CAD build for the part. Positions are in the model's coordinates, mm. A direction names the side the tool comes from. Round coordinates to 2 decimals unless told otherwise and drop trailing zeros. Write each loop counter-clockwise with the first axis right and the second up, starting at its lowest first coordinate (ties: lowest second). Pieces come first, ordered by that corner, then holes. Notation, with made-up numbers: (-30.75, 16) - (24.25, 16) arc R27 cw to (24.25, 38) - close; hole circle Ø6 at (87.25, -2.5). An arc over 180 degrees is marked (long way). Put each result on its own line as item: value. Start each with the question number.
Item 1: Drill centre lines: line 1 (X direction, y = 6.25, z = 34); line 2 (X direction, y = 14.3, z = 250); line 3 (Y direction, x = -5.5, z = 194). Where is each one in solid material? Low to high. Write a range as from..to.
Item 2: 3-axis set-ups, long thin cutter, end or side, ignore diameter. For faces 4 (the flat face through (0, -14, 138)), 5 (the flat face through (7.5, 0, 138)): which of +Z, -Z, +X, -X, +Y, -Y reach the whole face in a straight line?
Item 3: Mould opens along X. For faces 1 (the flat face through (-7.5, 0, 138)), 2 (the flat face through (0, 14, 138)), 3 (the flat face through (-7, 1, 0)) say: released by +X, released by -X, zero draft, split by the parting line, or undercut.
Item 4: Cut at B-B (y = 8.5). Give the cut face in (x, z), and give its area (3 significant figures).
Item 5: Cut at A-A (z = 223). Give the cut face in (x, y).
Autodesk Inventor part; units mm, degrees
ref_plane "YZ Plane" through (0, 0, 0) normal (1, 0, 0) x (0, 1, 0)
ref_plane "XZ Plane" through (0, 0, 0) normal (0, 1, 0) x (-1, 0, 0)
ref_plane "XY Plane" through (0, 0, 0) normal (0, 0, 1) x (1, 0, 0)
sketch "スケッチ1" plane through (0, 0, 0) normal (0, 0, 1) x (1, 0, 0)
  line L0 (7.5, 15) -> (-7.5, 15)
  line L1 (-7.5, 15) -> (-7.5, -15)
  line L2 (-7.5, -15) -> (7.5, -15)
  line L3 (7.5, -15) -> (7.5, 15)
  line L4 (7.5, 15) -> (-7.5, -15) construction
  line L5 (-7.5, 15) -> (7.5, -15) construction
  line L6 (-6.5, 14) -> (6.5, 14)
  line L7 (6.5, 14) -> (6.5, -14)
  line L8 (6.5, -14) -> (-6.5, -14)
  line L9 (-6.5, -14) -> (-6.5, 14)
  point P0 (0, 0)
  dimension "d0" = 15
  dimension "d1" = 30
  dimension "d2" = 1
extrude "押し出し1" add sketch "スケッチ1" along normal blind 280
sketch "スケッチ2" plane through (-7.5, 15, 0) normal (0, 1, 0) x (1, 0, 0)
  circle A0 centre (7.5, -7.5) radius 1.6
  circle A1 centre (7.5, -37.5) radius 1.6
  circle A2 centre (7.5, -67.5) radius 1.6
  line L0 (15, 0) -> (0, 0)
  circle A3 centre (7.5, -270) radius 1.6
  circle A4 centre (7.5, -260) radius 1.6
  circle A5 centre (7.5, -250) radius 1.6
  line L1 (15, -280) -> (0, -280)
  point P0 (7.5, 0)
  point P1 (7.5, 0)
  point P2 (7.5, -280)
  dimension "d5" = 3.2
  dimension "d6" = 3.2
  dimension "d7" = 3.2
  dimension "d8" = 7.5
  dimension "d9" = 30
  dimension "d10" = 30
  dimension "d11" = 3.2
  dimension "d12" = 3.2
  dimension "d13" = 3.2
  dimension "d14" = 10
  dimension "d15" = 10
  dimension "d16" = 10
extrude "押し出し2" cut sketch "スケッチ2" against normal through all
properties part number "アーム3_角柱1" material "アルミニウム 6061"
Output values:
1. line 1: -7.5..-6.5, 6.5..7.5
1. line 2: -7.5..-1.6, 1.6..7.5
1. line 3: -15..-14, 14..15
2. face 4: +Z, -Z
2. face 5: +Z, -Z, +X, +Y, -Y
3. face 1: released by -X
3. face 2: undercut
3. face 3: zero draft
4. outline: (-7.5, 0) - (-6.5, 0) - (-6.5, 280) - (-7.5, 280) - close; (6.5, 0) - (7.5, 0) - (7.5, 280) - (6.5, 280) - close
4. area: 560 mm2
5. outline: (-7.5, -15) - (7.5, -15) - (7.5, 15) - (-7.5, 15) - close; hole (-6.5, -14) - (6.5, -14) - (6.5, 14) - (-6.5, 14) - close
